```python
from build123d import *

# Parameters (mm, degrees)
SKETCH1_W            = 101.6
SKETCH1_H            = 47.8
BOSS_EXTRUDE1_DEPTH  = 76.2
SKETCH2_R            = 31.75
CUT_EXTRUDE1_DEPTH   = 95.648243512
FILLET1_R            = 3
LPATTERN1_COUNT      = 2
LPATTERN1_PITCH      = 82.55
LPATTERN1_COUNT_DIR2 = 2
LPATTERN1_PITCH_DIR2 = 40


with BuildPart() as part:
    # Sketch1 → Boss-Extrude1 (new body)
    with BuildSketch(Plane.XY):
        Rectangle(SKETCH1_W, SKETCH1_H)
    extrude(amount=BOSS_EXTRUDE1_DEPTH)

    # Sketch2 → Cut-Extrude1 (cut, through all)
    with BuildSketch(Plane.XY.offset(76.2)):
        with Locations((0, 26.9)):
            Circle(SKETCH2_R)
    extrude(amount=-CUT_EXTRUDE1_DEPTH, mode=Mode.SUBTRACT)

    # Fillet1
    fillet1_edges = [part.edges().sort_by_distance(p)[0] for p in [
        (-41.203974975, 23.9, 0),
        (-41.203974975, 23.9, 76.2),
        (0, -4.85, 76.2),
        (0, -4.85, 0),
        (31.607949949, 23.9, 38.1),
        (-31.607949949, 23.9, 38.1),
        (41.203974975, 23.9, 0),
        (-50.8, 23.9, 38.1),
        (50.8, 23.9, 38.1),
        (41.203974975, 23.9, 76.2),
    ]]
    fillet(fillet1_edges, radius=FILLET1_R)

    # Sketch4 → CBORE for 1/4 Binding Head Machine Screw1 (revolve, cut)
    with BuildSketch(Plane(origin=(-41.27, -23.9, 58.1), x_dir=(0, 0, -1), z_dir=(1, 0, 0))):
        Polygon((0, 0), (0, 47.8), (3.3782, 47.8), (3.3782, 4.191), (7.14375, 4.191), (7.14375, 0.532828266), (7.77875, 0), align=None)
    cbore_for_1_4_binding_head_machine_screw = revolve(axis=Axis((-41.27, -30.25, 58.1), (0, 1, 0)), mode=Mode.SUBTRACT)

    # LPattern1: CBORE for 1_4 Binding Head Machine Screw 2 × 2
    with Locations(*[(i * LPATTERN1_PITCH, 0, -j * LPATTERN1_PITCH_DIR2) for i in range(LPATTERN1_COUNT) for j in range(LPATTERN1_COUNT_DIR2) if (i, j) != (0, 0)]):
        add(cbore_for_1_4_binding_head_machine_screw, mode=Mode.SUBTRACT)


solid = part.part
```
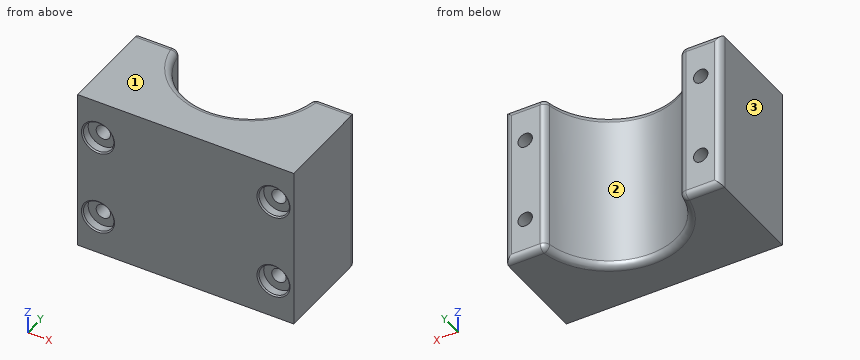
CAD build for the part. Positions are in the model's coordinates, mm. Face numbers are marked on the shaded views. Coordinates: 2 decimals unless noted, no trailing zeros. Order: outer loops, then holes, each group sorted by start corner. A loop starts at its lowest first (then second) coordinate and runs counter-clockwise, first axis right, second up. Notation, with made-up numbers: (-15, -5.75) - (0, -5.75) arc R26 cw to (0, 23.25) - close; hole circle Ø5 at (78, 15.5). An arc over 180 degrees is marked (long way). Use a Markdown table: item, result. Add a question column.
(1) Drill centre lines: line 1 along X through (y, z) = (-22, 58); line 2 along Z through (x, y) = (41, -22); line 3 along Z through (x, y) = (-41.27, 2.5). Where is each one in solid material? Low to high. Write a range as [from, to].
(2) Saw through at C-C (y = -9). Give the cut face in (x, z).
(3) Pull direction X, two halves, no side cores. Call the marked faces 1, 2 and 3: +X half, -X half, draft (parallel to the pull), parting line (faces both ways), or undercut.
(4) Saw through at B-B (z = 18.1). Count the separate pieces of the cut face and the enclosed holes in it, then the cut area to 3 significant figures.
(5) Saw through at A-A (x = 41.28). Give the cut face in (y, z), then the cut area to 3 significant figures.
(6) Flat gauge pin, fed straight in: pin 1 (23 mm diameter, centred on x = -41.27, z = 18.1, fed in from -Y). Where does the tip first touch, or does it go through?
(7) Saw through at D-D (z = 5). Give the cut face in (x, y), then the cut area to 3 significant figures.
Solved:
| question | item | result |
|---|---|---|
| 1 | line 1 | x = [-50.8, -48.41], [-34.13, 34.14], [48.42, 50.8] |
| 1 | line 2 | z = [0, 10.96], [25.24, 50.96], [65.24, 76.2] |
| 1 | line 3 | z = [0, 14.72], [21.48, 54.72], [61.48, 76.2] |
| 2 | outline | (-50.8, 0) - (50.8, 0) - (50.8, 76.2) - (-50.8, 76.2) - close; hole circle Ø6.76 at (-41.27, 18.1); hole circle Ø6.76 at (-41.27, 58.1); hole circle Ø6.76 at (41.28, 18.1); hole circle Ø6.76 at (41.28, 58.1) |
| 3 | face 1 | draft |
| 3 | face 2 | undercut |
| 3 | face 3 | -X half |
| 4 | separate pieces | 3 |
| 4 | enclosed holes | 0 |
| 4 | area | 2,750 mm² |
| 5 | outline | (-23.9, 0) - (20.9, 0) arc R3 ccw to (23.9, 3) - (23.9, 14.72) - (-19.71, 14.72) - (-19.71, 10.96) - (-23.37, 10.96) - (-23.9, 10.32) - close; (-23.9, 25.88) - (-23.37, 25.24) - (-19.71, 25.24) - (-19.71, 21.48) - (23.9, 21.48) - (23.9, 54.72) - (-19.71, 54.72) - (-19.71, 50.96) - (-23.37, 50.96) - (-23.9, 50.32) - close; (-23.9, 65.88) - (-23.37, 65.24) - (-19.71, 65.24) - (-19.71, 61.48) - (23.9, 61.48) - (23.9, 73.2) arc R3 ccw to (20.9, 76.2) - (-23.9, 76.2) - close |
| 5 | area | 2,930 mm² |
| 6 | pin 1 | stops at y = -23.9 |
| 7 | outline | (-50.8, -23.9) - (50.8, -23.9) - (50.8, 20.9) arc R3 ccw to (47.8, 23.9) - (34.23, 23.9) arc R3 ccw to (31.27, 21.42) arc R31.75 cw to (-31.27, 21.42) arc R3 ccw to (-34.23, 23.9) - (-47.8, 23.9) arc R3 ccw to (-50.8, 20.9) - close |
| 7 | area | 3,460 mm² |
